Can you work these out from the drawing? Everything is in mm from the part's minimum corner. Coordinates: 2 decimals unless noted, no trailing zeros. Loops run counter-clockwise (first coordinate to the right, second up) from the corner with the lowest first, then second, coordinate; pieces in that order, holes last. Notation, with made-up numbers: (-16, -17) - (18, -17) arc R17 ccw to (18, -8) - close; hole circle Ø8 at (-17.75, 9). An arc over 180 degrees is marked (long way). Use CSV: the item, a comma, the result in double quotes.
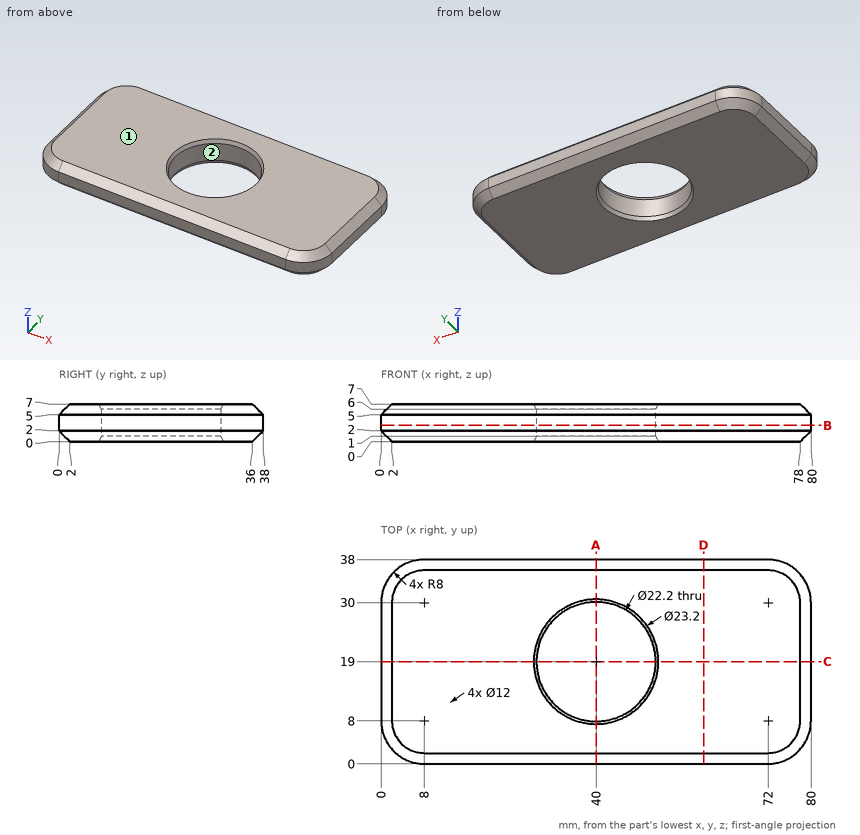
(1) Will these pins go through, and if not, where does the flat tip stop? pin 1 (4 mm diameter, centred on x = 25, z = 3.5, fed in from -Y); pin 2 (3 mm diameter, centred on x = 47.5, y = 21, fed in from +Z); pin 3 (3 mm diameter, centred on y = 4, z = 5, fed in from -X).
Computed:
pin 1,"stops at y = 0"
pin 2,"passes through"
pin 3,"stops at x = 0.4"
(2) Suppose I cut it at C-C (y = 19). Write out the boundary of the cut face in (x, z).
Computed:
outline,"(0, 2) - (2, 0) - (28.4, 0) - (28.9, 1) - (28.9, 6) - (28.4, 7) - (2, 7) - (0, 5) - close; (51.1, 1) - (51.6, 0) - (78, 0) - (80, 2) - (80, 5) - (78, 7) - (51.6, 7) - (51.1, 6) - close"
(3) Suppose I cut it at B-B (z = 3). Write out the boundary of the cut face in (x, y), plus the area to 3 significant figures.
Computed:
outline,"(0, 8) arc R8 ccw to (8, 0) - (72, 0) arc R8 ccw to (80, 8) - (80, 30) arc R8 ccw to (72, 38) - (8, 38) arc R8 ccw to (0, 30) - close; hole circle Ø22.2 at (40, 19)"
area,"2,600 mm²"
(4) Please list where these lines run through material, in increasing order: line 1 (Y direction, x = 40, z = 2.15); line 2 (Y direction, x = 42, z = 5.5); line 3 (X direction, y = 10, z = 6.75).
Computed:
line 1,"y = 0 to 7.9, 30.1 to 38"
line 2,"y = 0.5 to 8.08, 29.92 to 37.5"
line 3,"x = 1.75 to 32.88, 47.12 to 78.25"
(5) Thinking about a two-plate mould opening in Y: for the marked faces 1 and 2, which applies, +Y half, -Y half, draft (parallel to the pull), parting line (faces both ways), or undercut?
Computed:
face 1,"draft"
face 2,"undercut"
(6) Suppose I cut it at D-D (x = 60). Write out the boundary of the cut face in (y, z), plus the area to 3 significant figures.
Computed:
outline,"(0, 2) - (2, 0) - (36, 0) - (38, 2) - (38, 5) - (36, 7) - (2, 7) - (0, 5) - close"
area,"258 mm²"
(7) Suppose I cut it at A-A (x = 40). Write out the boundary of the cut face in (y, z).
Computed:
outline,"(0, 2) - (2, 0) - (7.4, 0) - (7.9, 1) - (7.9, 6) - (7.4, 7) - (2, 7) - (0, 5) - close; (30.1, 1) - (30.6, 0) - (36, 0) - (38, 2) - (38, 5) - (36, 7) - (30.6, 7) - (30.1, 6) - close"
